Geometry check sheet. Reference: the model listing, model coordinates, mm. Give positions to 0.01 mm unless a question says otherwise; leave off trailing zeros. Write each loop counter-clockwise with the first axis right and the second up, starting at its lowest first coordinate (ties: lowest second). Pieces come first, ordered by that corner, then holes. Notation, with made-up numbers: M 15.25,11.5 L 28.25,11.5 A27 ccw 28.25,50.5 Z; hole C -22,23.5 d8. An arc over 180 degrees is marked long. Use one line per item in the form item = value. Start each with the question number.
```python
from build123d import *

# Parameters (mm, degrees)
BOSS_EXTRUDE1_DEPTH     = 10
FILLET1_R               = 10
BOSS_EXTRUDE2_DEPTH     = 10
SKETCH3_R               = 2.75
CUT_EXTRUDE1_DEPTH      = 295.996739323
CUT_EXTRUDE2_DEPTH      = 295.996739323
CUT_EXTRUDE2_DEPTH_BACK = 295.996739323
SKETCH5_R               = 2.75
BOSS_EXTRUDE3_DEPTH     = 10
FILLET2_R               = 10
CUT_EXTRUDE3_DEPTH      = 10
SKETCH9_R               = 2.75
CUT_EXTRUDE4_DEPTH      = 387.134691526
SKETCH10_R              = 2.75
CUT_EXTRUDE5_DEPTH      = 387.134691526
CUT_EXTRUDE6_DEPTH      = 387.134691526
CUT_EXTRUDE6_DEPTH_BACK = 387.134691526
SKETCH11_R              = 2.75


with BuildPart() as part:
    # Sketch1 → Boss-Extrude1 (new body)
    with BuildSketch(Plane.XY):
        Polygon((75, -4.903810568), (0, 125), (0, 250), (-20, 250), (-20, 119.641016151), (57.679491924, -14.903810568), align=None)
        Polygon((0, 250), (0, 125), (75, -4.903810568), (92.320508076, 5.096189432), (20, 130.358983849), (20, 250), align=None)
    extrude(amount=BOSS_EXTRUDE1_DEPTH)

    # Fillet1
    fillet1_edges = [part.edges().sort_by_distance(p)[0] for p in [
        (57.679491924, -14.903810568, 5),
        (-20, 119.641016151, 5),
        (20, 130.358983849, 5),
    ]]
    fillet(fillet1_edges, radius=FILLET1_R)

    # Sketch2 → Boss-Extrude2 (add)
    with BuildSketch(Plane.XY.offset(10)):
        with BuildLine():
            Line((0, 250), (20, 250))
            Line((20, 250), (20, 260))
            ThreePointArc((20, 260), (0, 280), (-20, 260))
            Line((-20, 260), (-20, 250))
            Line((-20, 250), (0, 250))
        make_face()
        with BuildLine():
            ThreePointArc((0, 264), (4, 260), (0, 256))
            ThreePointArc((0, 256), (-4, 260), (0, 264))
        make_face(mode=Mode.SUBTRACT)
    extrude(amount=-BOSS_EXTRUDE2_DEPTH)

    # Sketch3 → Cut-Extrude1 (cut, through all)
    with BuildSketch(Plane.XY.offset(10)):
        with Locations((0, 190)):
            Circle(SKETCH3_R)
        with Locations((0, 225)):
            Circle(SKETCH3_R)
    extrude(amount=-CUT_EXTRUDE1_DEPTH, mode=Mode.SUBTRACT)

    # Sketch5 → Cut-Extrude2 (cut, two sides: drawn at the far end of the back side and taken through both)
    with BuildSketch(Plane.XY.offset(10).offset(-CUT_EXTRUDE2_DEPTH_BACK)):
        with Locations((60, 21.076951546)):
            Circle(SKETCH5_R)
        with Locations((70, 3.75644347)):
            Circle(SKETCH5_R)
    extrude(amount=CUT_EXTRUDE2_DEPTH + CUT_EXTRUDE2_DEPTH_BACK, mode=Mode.SUBTRACT)

    # Sketch7 → Boss-Extrude3 (add)
    with BuildSketch(Plane.XY.offset(10)):
        with BuildLine():
            ThreePointArc((-14.142135624, 245.857864376), (-14.142135624, 274.142135624), (14.142135624, 274.142135624))
            Line((14.142135624, 274.142135624), (-105.857864376, 394.142135624))
            ThreePointArc((-105.857864376, 394.142135624), (-134.142135624, 394.142135624), (-134.142135624, 365.857864376))
            Line((-134.142135624, 365.857864376), (-14.142135624, 245.857864376))
        make_face()
    extrude(amount=-BOSS_EXTRUDE3_DEPTH)

    # Fillet2
    fillet2_edges = [part.edges().sort_by_distance(p)[0] for p in [
        (-20, 251.715728753, 5),
    ]]
    fillet(fillet2_edges, radius=FILLET2_R)

    # Sketch8 → Cut-Extrude3 (cut)
    with BuildSketch(Plane.XY.offset(10)):
        with BuildLine():
            ThreePointArc((-104.142135624, 335.857864376), (-104.142135624, 364.142135624), (-75.857864376, 364.142135624))
            Line((-75.857864376, 364.142135624), (-105.857864376, 394.142135624))
            ThreePointArc((-105.857864376, 394.142135624), (-134.142135624, 394.142135624), (-134.142135624, 365.857864376))
            Line((-134.142135624, 365.857864376), (-104.142135624, 335.857864376))
        make_face()
    extrude(amount=-CUT_EXTRUDE3_DEPTH, mode=Mode.SUBTRACT)

    # Sketch9 → Cut-Extrude4 (cut, through all)
    with BuildSketch(Plane.XY.offset(10)):
        with Locations((-90, 350)):
            Circle(SKETCH9_R)
        with Locations((-68.786796564, 328.786796564)):
            Circle(SKETCH9_R)
    extrude(amount=-CUT_EXTRUDE4_DEPTH, mode=Mode.SUBTRACT)

    # Sketch10 → Cut-Extrude5 (cut, through all)
    with BuildSketch(Plane.XY.offset(10)):
        with Locations((40, 55.717967697)):
            Circle(SKETCH10_R)
    extrude(amount=-CUT_EXTRUDE5_DEPTH, mode=Mode.SUBTRACT)

    # Sketch11 → Cut-Extrude6 (cut, two sides: drawn at the far end of the back side and taken through both)
    with BuildSketch(Plane.XY.offset(10).offset(-CUT_EXTRUDE6_DEPTH_BACK)):
        with Locations((0.340741737, 145.091301473)):
            Circle(SKETCH11_R)
        with Locations((0.340741737, 125.091301473)):
            Circle(SKETCH11_R)
        with Locations((10.340741737, 107.770793398)):
            Circle(SKETCH11_R)
    extrude(amount=CUT_EXTRUDE6_DEPTH + CUT_EXTRUDE6_DEPTH_BACK, mode=Mode.SUBTRACT)


solid = part.part
```
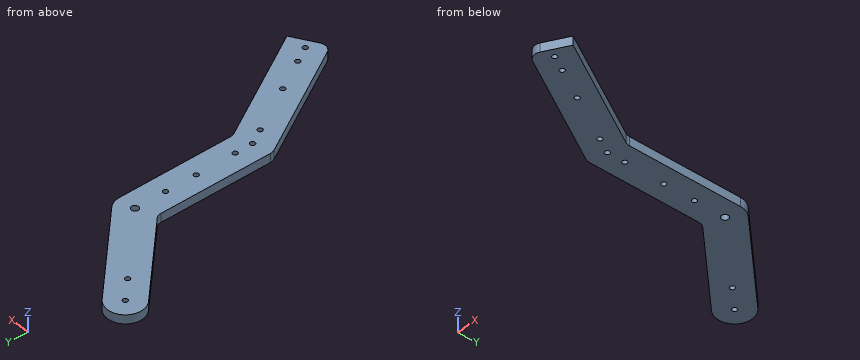
(1) Depth check by flat-ended pin: pin 1 (4.5 mm diameter, centred on x = 40, y = 55.72, fed in from +Z); pin 2 (6 mm diameter, centred on y = 275, z = 5.5, fed in from -X); pin 3 (4 mm diameter, centred on x = -37.5, z = 1.5, fed in from +Y); pin 4 (1.5 mm diameter, centred on y = 255.5, z = 8.5, fed in from +X). Enter the tip coordinate at first touch or a pass-through.
(2) Sectioned sample at C-C, the plane x = -36. Record the boundary of the cut face in (y, z).
(3) Thickness scan on probe 1 along X at (y, z) = (190, 7.75); probe 2 along X at (y, z) = (193.5, 2); probe 3 along Y at (x, z) = (60, 3). Record the ranges inside material, lowest first. Write a range as [from, to].
(4) Sectioned sample at B-B, the plane y = 233. Record the boundary of the cut face in (x, z), plus the area to 3 significant figures.
(5) Sectioned sample at A-A, the plane z = 2. State how many separate pieces and enclosed holes the cut face has, plus the area to 3 significant figures.
Numbers:
q1.pin_1 = through
q1.pin_2 = -46.28
q1.pin_3 = 327.78
q1.pin_4 = 20
q2.outline = M 267.72,0 L 324.28,0 L 324.28,10 L 267.72,10 Z
q3.probe_1 = [-20, -2.75], [2.75, 20]
q3.probe_2 = [-20, 20]
q3.probe_3 = [-11.15, 18.33], [23.83, 61.08]
q4.outline = M -20,0 L 20,0 L 20,10 L -20,10 Z
q4.area = 400 mm2
q5.separate_pieces = 1
q5.enclosed_holes = 11
q5.area = 16,800 mm2
